Work out the finished part from the listing and answer in its coordinate system (mm). Face numbers are marked on the shaded views. A direction names the side the tool comes from. Give positions to 0.01 mm unless a question says otherwise; leave off trailing zeros. Use a Markdown table: item, result. Add a question column.
```python
from build123d import *

# Parameters (mm, degrees)
CORTAR_EXTRUIR1_DEPTH                       = 36.08204683
CORTAR_EXTRUIR1_DEPTH_BACK                  = 36.08204683
CROQUIS3_W                                  = 4
CROQUIS3_H                                  = 3.25
CORTAR_EXTRUIR2_DEPTH                       = 36.08204683
CORTAR_EXTRUIR3_DEPTH                       = 38.983549135
CORTAR_EXTRUIR3_DEPTH_BACK                  = 38.983549135
SALIENTE_EXTRUIR1_DEPTH                     = 2.5
SALIENTE_EXTRUIR1_DEPTH_BACK                = 2.5
CROQUIS9_W                                  = 3
CROQUIS9_H                                  = 7
CORTAR_EXTRUIR5_DEPTH                       = 42.865857269
CORTAR_EXTRUIR6_DEPTH                       = 6.5
CROQUIS12_R                                 = 4.45
CORTAR_EXTRUIR7_DEPTH                       = 6.5
CORTAR_EXTRUIR7_DEPTH_BACK                  = 6.5
SALIENTE_EXTRUIR2_REACH                     = 65.166
SALIENTE_EXTRUIR2_END_RADIUS                = 4.45
CROQUIS13_R                                 = 1
CORTAR_EXTRUIR8_DEPTH                       = 42.865857349
DI_METRO_DE_TALADRO_1_0_1_1_D               = 1
DI_METRO_DE_TALADRO_1_0_1_1_DEPTH           = 2
DI_METRO_DE_TALADRO_1_0_1_1_TIP             = 0.30043031
DI_METRO_DE_TALADRO_1_0_1_1_ON_FACE_2_D     = 1
DI_METRO_DE_TALADRO_1_0_1_1_ON_FACE_2_DEPTH = 2
DI_METRO_DE_TALADRO_1_0_1_1_ON_FACE_2_TIP   = 0.30043031
CORTAR_EXTRUIR9_START                       = -2.5
CROQUIS16_W                                 = 2
CROQUIS16_H                                 = 7
CORTAR_EXTRUIR9_DEPTH                       = 2.5


with BuildPart() as part:
    # Croquis1 → Revolución1 (revolve)
    with BuildSketch(Plane.XY, mode=Mode.PRIVATE) as revoluci_n1_sk:
        with BuildLine():
            Line((18, 0), (21, 0))
            Line((21, 0), (21, 0.5))
            Line((21, 0.5), (23, 0.5))
            Line((23, 0.5), (24.331419138, 2.25))
            ThreePointArc((24.331419138, 2.25), (24.5, 2.75), (24.331419138, 3.25))
            Line((24.331419138, 3.25), (23, 5))
            Line((23, 5), (19.5, 5))
            Line((19.5, 5), (19.5, 5.5))
            Line((19.5, 5.5), (19, 5.5))
            Line((19, 5.5), (19, 4.75))
            Line((19, 4.75), (18, 4.75))
            Line((18, 4.75), (18, 4.5))
            Line((18, 4.5), (21.5, 4.5))
            Line((21.5, 4.5), (21.5, 1))
            Line((21.5, 1), (18, 1))
            Line((18, 1), (18, 0))
        make_face()
    revolve(revoluci_n1_sk.sketch.rotate(Axis((0, 0, 0), (0, 1, 0)), 90), axis=Axis((0, 0, 0), (0, 1, 0)))

    # Croquis2 → Cortar-Extruir1 (cut, two sides)
    with BuildSketch(Plane(origin=(0, 0, 0), x_dir=(0, 0, -1), z_dir=(1, 0, 0))) as cortar_extruir1_sk:
        with BuildLine():
            Line((23, 3), (23, 5))
            Line((23, 5), (24.5, 5))
            Line((24.5, 5), (24.5, 2.5))
            Line((24.5, 2.5), (23.5, 2.5))
            ThreePointArc((23.5, 2.5), (23.146446609, 2.646446609), (23, 3))
        make_face()
    extrude(amount=CORTAR_EXTRUIR1_DEPTH, mode=Mode.SUBTRACT)
    extrude(cortar_extruir1_sk.sketch, amount=-CORTAR_EXTRUIR1_DEPTH_BACK, mode=Mode.SUBTRACT)

    # Croquis3 → Cortar-Extruir2 (cut, through all)
    with BuildSketch(Plane.XZ):
        with Locations((0, 19.125)):
            Rectangle(CROQUIS3_W, CROQUIS3_H)
    extrude(amount=-CORTAR_EXTRUIR2_DEPTH, mode=Mode.SUBTRACT)

    # Croquis5 → Revolución2 (revolve)
    with BuildSketch(Plane(origin=(0, 0, 0), x_dir=(0, 0, -1), z_dir=(1, 0, 0))):
        Polygon((-22, 0.25), (-22, 2.75), (-28.5, 2.75), (-28.5, 0.25), (-28, 0.25), (-27.5, 0.75), (-27, 0.25), (-26.5, 0.25), (-26.25, 0.5), (-26, 0.25), align=None)
    revolve(axis=Axis((0, 2.75, 28.5), (0, 0, -1)))

    # Croquis6 → Cortar-Extruir3 (cut, two sides)
    with BuildSketch(Plane(origin=(0, 0, 0), x_dir=(0, 0, -1), z_dir=(1, 0, 0))) as cortar_extruir3_sk:
        Polygon((-22, 0), (-22, 0.5), (-25.75, 0.5), (-26.25, 0), (-26.25, -0.75), (-22, -0.75), align=None)
        Polygon((-22, 5), (-25.75, 5), (-26.25, 5.5), (-26.25, 6.25), (-22, 6.25), (-22, 5.5), align=None)
        Polygon((-28, 5.25), (-28.5, 4.75), (-28.5, 5.25), align=None)
        Polygon((-28, 0.25), (-28.5, 0.75), (-28.5, 0.25), align=None)
    extrude(amount=CORTAR_EXTRUIR3_DEPTH, mode=Mode.SUBTRACT)
    extrude(cortar_extruir3_sk.sketch, amount=-CORTAR_EXTRUIR3_DEPTH_BACK, mode=Mode.SUBTRACT)

    # Croquis8 → Saliente-Extruir1 (add, two sides)
    with BuildSketch(Plane(origin=(0, 2.75, 0), x_dir=(-1, 0, 0), z_dir=(0, 1, 0))) as saliente_extruir1_sk:
        with BuildLine():
            ThreePointArc((-7.261843774, 30.375), (0, 27.25), (7.261843774, 30.375))
            ThreePointArc((7.261843774, 30.375), (0, 33.5), (-7.261843774, 30.375))
        make_face()
    extrude(amount=SALIENTE_EXTRUIR1_DEPTH)
    extrude(saliente_extruir1_sk.sketch, amount=-SALIENTE_EXTRUIR1_DEPTH_BACK)

    # Croquis9 → Cortar-Extruir5 (cut, through all)
    with BuildSketch(Plane(origin=(0, 0, 0), x_dir=(1, 0, 0), z_dir=(0, 1, 0))):
        with Locations((6.5, -29.5)):
            Rectangle(CROQUIS9_W, CROQUIS9_H)
        with Locations((-6.5, -29.5)):
            Rectangle(CROQUIS9_W, CROQUIS9_H)
    extrude(amount=CORTAR_EXTRUIR5_DEPTH, mode=Mode.SUBTRACT)

    # Croquis10 → Cortar-Extruir6 (cut)
    with BuildSketch(Plane.XY.offset(33.5)):
        with BuildLine():
            Line((5, 5.25), (0, 5.25))
            ThreePointArc((0, 5.25), (2.610076627, 4.866922091), (5, 3.75))
            Line((5, 3.75), (5, 5.25))
        make_face()
        with BuildLine():
            Line((-5, 5.25), (-5, 3.75))
            ThreePointArc((-5, 3.75), (-2.610076627, 4.866922091), (0, 5.25))
            Line((0, 5.25), (-5, 5.25))
        make_face()
        with BuildLine():
            ThreePointArc((0, 0.25), (-2.610076627, 0.633077909), (-5, 1.75))
            Line((-5, 1.75), (-5, 0.25))
            Line((-5, 0.25), (0, 0.25))
        make_face()
        with BuildLine():
            ThreePointArc((5, 1.75), (2.610076627, 0.633077909), (0, 0.25))
            Line((0, 0.25), (5, 0.25))
            Line((5, 0.25), (5, 1.75))
        make_face()
    extrude(amount=-CORTAR_EXTRUIR6_DEPTH, mode=Mode.SUBTRACT)

    # Croquis12 → Cortar-Extruir7 (cut, two sides)
    with BuildSketch(Plane(origin=(0, 2.75, 0), x_dir=(-1, 0, 0), z_dir=(0, 1, 0))) as cortar_extruir7_sk:
        with Locations((0.113074667, 35.198563152)):
            Circle(CROQUIS12_R)
    extrude(amount=CORTAR_EXTRUIR7_DEPTH, mode=Mode.SUBTRACT)
    extrude(cortar_extruir7_sk.sketch, amount=-CORTAR_EXTRUIR7_DEPTH_BACK, mode=Mode.SUBTRACT)

    # Saliente-Extruir2: up to this cylinder (the profile starts inside it)
    saliente_extruir2_end = Plane(origin=(-0.113074667, 2.75, 35.198563152), z_dir=(0, -1, 0)) * Cylinder(SALIENTE_EXTRUIR2_END_RADIUS, 140.232, mode=Mode.PRIVATE)
    # Croquis15 → Saliente-Extruir2 (add, up to the surface)
    with BuildSketch(Plane.XY.offset(33.5), mode=Mode.PRIVATE) as saliente_extruir2_sk1:
        with BuildLine():
            Line((-1, 3.868033989), (1, 3.868033989))
            ThreePointArc((1, 3.868033989), (1.5, 2.75), (1, 1.631966011))
            Line((1, 1.631966011), (-1, 1.631966011))
            ThreePointArc((-1, 1.631966011), (-1.5, 2.75), (-1, 3.868033989))
        make_face()
    saliente_extruir2_tool1 = extrude(saliente_extruir2_sk1.sketch, amount=-SALIENTE_EXTRUIR2_REACH, mode=Mode.PRIVATE) & saliente_extruir2_end
    add(saliente_extruir2_tool1.solids().sort_by_distance((0, 2.75, 33.5))[0])

    # Croquis13 → Cortar-Extruir8 (cut, through all)
    with BuildSketch(Plane.XY):
        with Locations(Location((0, 2.75, 0), (0, 0, 180))):
            Circle(CROQUIS13_R)
    extrude(amount=CORTAR_EXTRUIR8_DEPTH, mode=Mode.SUBTRACT)

    # Diámetro de taladro Ø1.0 (1)1
    with Locations(Plane(origin=(5, 2.75, 30.375), x_dir=(0, 0, 1), z_dir=(1, 0, 0))):
        with Locations((0, 0)):
            Hole(DI_METRO_DE_TALADRO_1_0_1_1_D / 2, depth=DI_METRO_DE_TALADRO_1_0_1_1_DEPTH)
            with Locations((0, 0, -(DI_METRO_DE_TALADRO_1_0_1_1_DEPTH + DI_METRO_DE_TALADRO_1_0_1_1_TIP / 2))):  # 118° drill point
                Cone(0, DI_METRO_DE_TALADRO_1_0_1_1_D / 2, DI_METRO_DE_TALADRO_1_0_1_1_TIP, mode=Mode.SUBTRACT)

    # Diámetro de taladro Ø1.0 (1)1 on face 2
    with Locations(Plane(origin=(-5, 2.75, 30.375), x_dir=(0, 0, -1), z_dir=(-1, 0, 0))):
        with Locations((0, 0)):
            Hole(DI_METRO_DE_TALADRO_1_0_1_1_ON_FACE_2_D / 2, depth=DI_METRO_DE_TALADRO_1_0_1_1_ON_FACE_2_DEPTH)
            with Locations((0, 0, -(DI_METRO_DE_TALADRO_1_0_1_1_ON_FACE_2_DEPTH + DI_METRO_DE_TALADRO_1_0_1_1_ON_FACE_2_TIP / 2))):  # 118° drill point
                Cone(0, DI_METRO_DE_TALADRO_1_0_1_1_ON_FACE_2_D / 2, DI_METRO_DE_TALADRO_1_0_1_1_ON_FACE_2_TIP, mode=Mode.SUBTRACT)

    # Croquis16 → Cortar-Extruir9 (cut)
    with BuildSketch(Plane(origin=(0, 5.5, 0), x_dir=(1, 0, 0), z_dir=(0, 1, 0)).offset(CORTAR_EXTRUIR9_START)):
        with Locations((0, 19.5)):
            Rectangle(CROQUIS16_W, CROQUIS16_H)
    extrude(amount=CORTAR_EXTRUIR9_DEPTH, mode=Mode.SUBTRACT)


solid = part.part
```
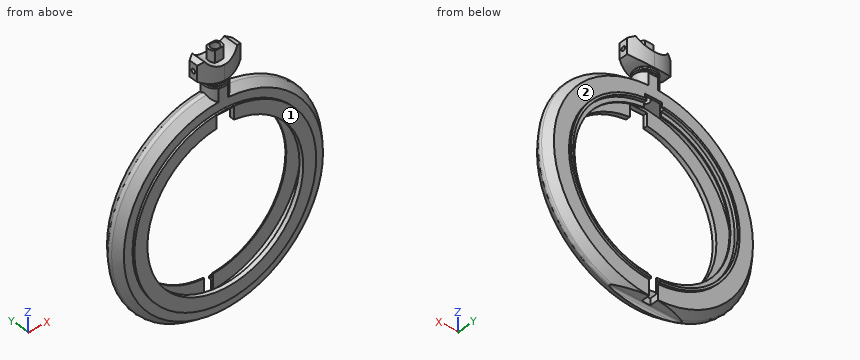
1) Which of the six approach directions +Z, -Z, +X, -X, +Y, -Y give full straight-line access (tool end or side, diameter ignored) to the marked faces 1 and 2?
2) Flat-ended cylindrical pins translate along their axes: pin 1 (0.5 mm diameter, centred on y = 5, z = 19, fed in from +X); pin 2 (3 mm diameter, centred on x = -19, y = 2, fed in from +Z); pin 3 (4 mm diameter, centred on x = 12, z = 20.5, fed in from +Y). Find the tip coordinate at first contact, or state that the pin passes through.
3) Straight lines are drawn through the part: line 1 (X direction, y = 0.4, z = 0); line 2 (Z direction, x = -3.6, y = 2.75) (3 decimals); line 3 (Z direction, x = -1, y = 0.6). For each, find the intervals that lie inside material, in ascending order.
A:
| question | item | result |
|---|---|---|
| 1 | face 1 | +Z, -Z, +X, -X, -Y |
| 1 | face 2 | +Y |
| 2 | pin 1 | x = 13.45 |
| 2 | pin 2 | z = 17 |
| 2 | pin 3 | y = 5 |
| 3 | line 1 | -21 to -18, 18 to 21 |
| 3 | line 2 | -23.067 to -21.196, 21.196 to 24.234, 27.92 to 29.875, 30.875 to 32.434 |
| 3 | line 3 | -23.05 to -17.97, 20.75 to 26.13, 26.37 to 27.13, 27.3 to 30.84 |
